Geometry: final body of the model. Coordinates: model frame, mm. A direction names the side the tool comes from. Coordinates: 2 decimals unless noted, no trailing zeros. Write each loop counter-clockwise with the first axis right and the second up, starting at its lowest first coordinate (ties: lowest second). Pieces come first, ordered by that corner, then holes. Notation, with made-up numbers: M 37,-34 L 86,-34 A33 cw 86,-2 Z; hole C 56.5,49 d2. An arc over 180 degrees is marked long. Write item = value, one per line. Start each with the question number.
Item 1: Ray query, L1, parallel to Y at x = 0, z = 0.6; L2, parallel to Z at x = 8.5, y = -7; L3, parallel to Y at x = -3.75, z = 3. Return the intervals inside material, ascending. Write a range as [from, to].
Item 2: Section A-A on y = 0. Output: boundary loops of the cut face in (x, z).
Item 3: Reachability of faces 5 (the flat face through (-9, 7, 10)), 6 (the cylindrical face through (5.19, -9.98, 6.06)) from +Z, -Z, +X, -X, +Y, -Y: full face, straight path, thin tool, end or side. Return the list, or none.
Item 4: Pull-direction query (X, two-part tool) for faces 1 (the cylindrical face through (11.923, 3.755, 4.93)), 2 (the flat face through (-3, -5.4, 0)), 3 (the cylindrical face through (-6, 0, 1)), 4 (the flat face through (5, -5, 2)); classes: +X half, -X half, draft (parallel to the pull), parting line (faces both ways), or undercut.
Item 5: Section D-D on y = -9. Output: boundary loops of the cut face in (x, z).
Item 6: First-contact query: pin 1 Ø1 at (y, z) = (2.5, 6.5) entering from -X; pin 2 Ø5 at (y, z) = (-6.5, 7) entering from +X; pin 3 Ø6 at (y, z) = (-10, 8.5) entering from +X. Flat tips, straight axial feed; report the tip coordinate or a pass-through.
Item 7: Section C-C on z = 4.5. Output: boundary loops of the cut face in (x, y).
from build123d import *

# Parameters (mm, degrees)
F0_R     = 12.5
F1_DEPTH = 10
F2_R     = 6
F3_DEPTH = 25
F2_R_2   = 11.25
F4_DEPTH = 8


with BuildPart() as f1:
    # F0 (on Top) → F1 (new body)
    with BuildSketch(Plane.XY):
        Circle(F0_R)
    extrude(amount=F1_DEPTH)

    # F2 (on face) → F3 (cut)
    with BuildSketch(Plane.XY.offset(10)):
        Circle(F2_R)
    extrude(amount=-F3_DEPTH, mode=Mode.SUBTRACT)

    # F2 (on face) → F4 (cut)
    with BuildSketch(Plane.XY.offset(10)):
        Circle(F2_R_2)
        Circle(F2_R, mode=Mode.SUBTRACT)
    extrude(amount=-F4_DEPTH, mode=Mode.SUBTRACT)


solid = f1.part
Responses:
q1.L1 = [-12.5, -6], [6, 12.5]
q1.L2 = [0, 2]
q1.L3 = [-11.92, -10.61], [10.61, 11.92]
q2.outline = M -12.5,0 L -6,0 L -6,2 L -11.25,2 L -11.25,10 L -12.5,10 Z; M 6,0 L 12.5,0 L 12.5,10 L 11.25,10 L 11.25,2 L 6,2 Z
q3.face_5 = +Z, +X, -X, +Y, -Y
q3.face_6 = +Z
q4.face_1 = parting line
q4.face_2 = draft
q4.face_3 = undercut
q4.face_4 = undercut
q5.outline = M -8.67,0 L 8.67,0 L 8.67,10 L 6.75,10 L 6.75,2 L -6.75,2 L -6.75,10 L -8.67,10 Z
q6.pin_1 = -12.34
q6.pin_2 = 11.84
q6.pin_3 = 10.36
q7.outline = C 0,0 d25; hole C 0,0 d22.5
